Could you check a few things on this model? Use its own coordinates, in mm. Face numbers are marked on the shaded views. A direction names the side the tool comes from. Round coordinates to 2 decimals unless told otherwise and drop trailing zeros. Write each loop counter-clockwise with the first axis right and the second up, starting at its lowest first coordinate (ties: lowest second). Pieces come first, ordered by that corner, then holes. Notation, with made-up numbers: (3, 2.5) -> (54, 2.5) arc R21 cw to (54, 22.5) -> close; hole circle Ø2 at (-29, 30.25). An arc over 180 degrees is marked (long way). Answer in a Markdown table with one row per item. Add a question column.
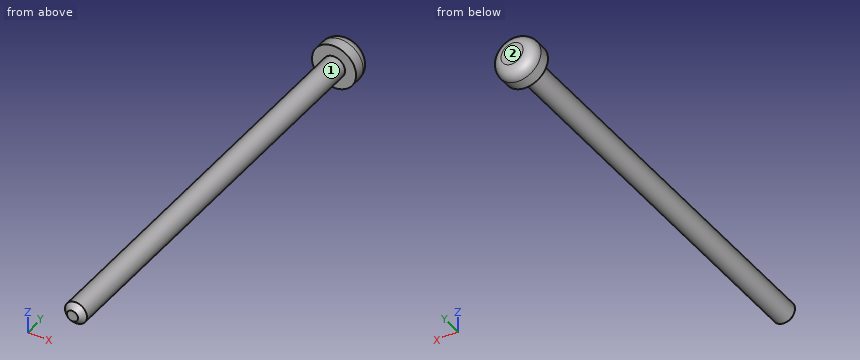
```python
from build123d import *

# Parameters (mm, degrees)
SKETCH1_R           = 2.032
BOSS_EXTRUDE1_DEPTH = 76.2
SKETCH2_R           = 4.064
BOSS_EXTRUDE2_DEPTH = 4.064
FILLET1_R           = 2.032
CHAMFER1_SIZE       = 1.016


with BuildPart() as part:
    # Sketch1 → Boss-Extrude1 (new body)
    with BuildSketch(Plane(origin=(0, 0, 0), x_dir=(1, 0, 0), z_dir=(0, 1, 0))):
        with Locations(Location((0, 0, 0), (0, 0, 90))):
            Circle(SKETCH1_R)
    extrude(amount=BOSS_EXTRUDE1_DEPTH)

    # Sketch2 → Boss-Extrude2 (add)
    with BuildSketch(Plane(origin=(0, 76.2, 0), x_dir=(1, 0, 0), z_dir=(0, 1, 0))):
        with Locations(Location((0, 0, 0), (0, 0, 270))):
            Circle(SKETCH2_R)
    extrude(amount=BOSS_EXTRUDE2_DEPTH)

    # Fillet1
    fillet1_edges = [part.edges().sort_by_distance(p)[0] for p in [
        (0, 80.264, -4.064),
    ]]
    fillet(fillet1_edges, radius=FILLET1_R)

    # Chamfer1
    chamfer1_edges = [part.edges().sort_by_distance(p)[0] for p in [
        (0, 0, 2.032),
    ]]
    chamfer(chamfer1_edges, length=CHAMFER1_SIZE)


solid = part.part
```
(1) On a 3-axis mill with a long thin cutter (end or side, diameter ignored), from which of +Z, -Z, +X, -X, +Y, -Y can I reach the whole of each face in a straight line? I mean the marked faces 1 and 2. Say none if no direction works.
(2) Suppose I cut it at A-A, the plane y = 42. Please give me the cut outline in (x, z), then the cut area to 3 significant figures.
(3) I need wall thicknesses on L1, parallel to X at y = 24, z = 0; L2, parallel to X at y = 76.5, z = 0.25; L3, parallel to Z at x = -0.25, y = 14. Which ranges of each line are inside material? Lowest first, please.
(4) For P1, Ø2, axis at y = 37.5, z = 0, coming from the +X side; P2, Ø4, axis at y = 10, z = -2, coming from the -X side, each with a flat end and sliding along its axis, tell me the tip position at first contact or that it passes through.
Response:
| question | item | result |
|---|---|---|
| 1 | face 1 | -Y |
| 1 | face 2 | +Z, -Z, +X, -X, +Y |
| 2 | outline | circle Ø4.06 at (0, 0) |
| 2 | area | 13.0 mm² |
| 3 | L1 | -2.03 to 2.03 |
| 3 | L2 | -4.06 to 4.06 |
| 3 | L3 | -2.02 to 2.02 |
| 4 | P1 | x = 2.03 |
| 4 | P2 | x = -2.03 |
